Read the model definition and answer for the solid it produces. Units are mm, in the model's axes. Face numbers are marked on the shaded views. A direction names the side the tool comes from. Coordinates: 2 decimals unless noted, no trailing zeros. Write each loop counter-clockwise with the first axis right and the second up, starting at its lowest first coordinate (ties: lowest second). Pieces come first, ordered by that corner, then holes. Notation, with made-up numbers: (41.5, 53) - (70.5, 53) arc R11 cw to (70.5, 61) - close; hole circle Ø7 at (29, -23). An arc over 180 degrees is marked (long way). Use a Markdown table: item, result.
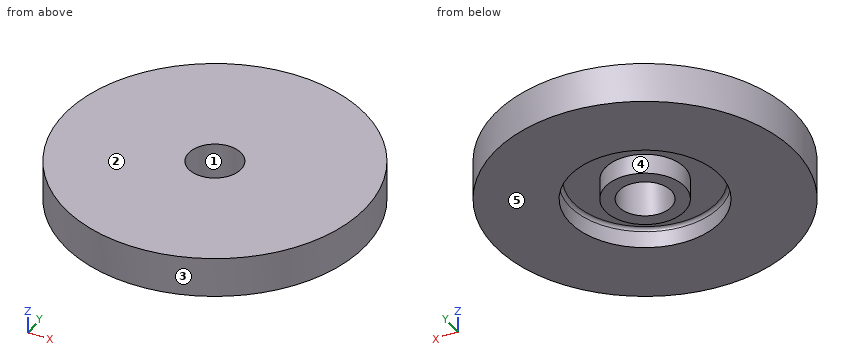
from build123d import *

# Parameters (mm, degrees)
SKETCH_1_R          = 150
SKETCH_1_R_2        = 75
SKETCH_1_R_3        = 38.1
EXTRUDE_1_DEPTH     = 40
SKETCH_1_4_R        = 75
SKETCH_1_4_R_2      = 38.1
CUT_EXTRUDE_1_DEPTH = 20
FILLET_1_R          = 3.2
SCALE_1_SCALE       = 0.4
SKETCH_3_R          = 15.813682359
SKETCH_3_R_2        = 10.461949065
EXTRUDE_2_DEPTH     = 16


with BuildPart() as part:
    # 草图1 → 凸台-拉伸1 (new body)
    # profile 1 of 2: a face of its own
    with BuildSketch(Plane.XY):
        Circle(SKETCH_1_R)
        Circle(SKETCH_1_R_2, mode=Mode.SUBTRACT)
    # profile 2 of 2: a face of its own
    with BuildSketch(Plane.XY):
        Circle(SKETCH_1_R_2)
        Circle(SKETCH_1_R_3, mode=Mode.SUBTRACT)
    extrude(amount=EXTRUDE_1_DEPTH)

    # 草图1<4> → 切除-拉伸1 (cut)
    with BuildSketch(Plane.XY):
        Circle(SKETCH_1_4_R)
        Circle(SKETCH_1_4_R_2, mode=Mode.SUBTRACT)
    extrude(amount=CUT_EXTRUDE_1_DEPTH, mode=Mode.SUBTRACT)

    # 圆角1
    fillet_1_edges = [part.edges().sort_by_distance(p)[0] for p in [
        (-75, 0, 20),
    ]]
    fillet(fillet_1_edges, radius=FILLET_1_R)


with BuildPart() as part_1:
    # 缩放比例1: scaled about (0, 0, 21.099696872)
    add(part.part.scale(SCALE_1_SCALE).moved(Location((0, 0, 12.659818123))))

    # 草图3 → 凸台-拉伸2 (add)
    with BuildSketch(Plane.XY.offset(28.659818123)):
        Circle(SKETCH_3_R)
        Circle(SKETCH_3_R_2, mode=Mode.SUBTRACT)
    extrude(amount=-EXTRUDE_2_DEPTH)


solid = part_1.part
(1) The mould has two halves that part along X. Classify the marked faces 1, 2 and 3: pulls with the +X half, pulls with the -X half, needs draft (parallel to the pull), parting line crosses it, or undercut.
Report:
| item | result |
|---|---|
| face 1 | undercut |
| face 2 | needs draft |
| face 3 | parting line crosses it |
(2) A cutting plane is placed at A-A, the plane x = 0. Write down the section's boundary in (y, z).
Report:
| item | result |
|---|---|
| outline | (-60, 12.66) - (-30, 12.66) - (-30, 19.38) arc R1.28 cw to (-28.72, 20.66) - (-15.81, 20.66) - (-15.81, 12.66) - (-10.46, 12.66) - (-10.46, 28.66) - (-60, 28.66) - close; (10.46, 12.66) - (15.81, 12.66) - (15.81, 20.66) - (28.72, 20.66) arc R1.28 cw to (30, 19.38) - (30, 12.66) - (60, 12.66) - (60, 28.66) - (10.46, 28.66) - close |
(3) Straight lines are drawn through the part: L1, parallel to Y at x = 0, z = 16; L2, parallel to X at y = -14.5, z = 14.25; L3, parallel to Y at x = -16, z = 18.25. For each, find the intervals that lie inside material, in ascending order.
Report:
| item | result |
|---|---|
| L1 | y = -60 to -30, -15.81 to -10.46, 10.46 to 15.81, 30 to 60 |
| L2 | x = -58.22 to -26.26, -6.31 to 6.31, 26.26 to 58.22 |
| L3 | y = -57.83 to -25.38, 25.38 to 57.83 |
(4) A cutting plane is placed at C-C, the plane z = 17.5. Write down the section's boundary in (x, y).
Report:
| item | result |
|---|---|
| outline | circle Ø120 at (0, 0); circle Ø31.63 at (0, 0); hole circle Ø60 at (0, 0); hole circle Ø20.92 at (0, 0) |
(5) For the marked faces 4 and 5, determine the directions among +Z, -Z, +X, -X, +Y, -Y from which every point of the face is accessible in a straight line to the end or side of a thin tool.
Report:
| item | result |
|---|---|
| face 4 | -Z |
| face 5 | -Z, +X, -X, +Y, -Y |
(6) Each of these flat-tipped pins is pushed along its axis until it touches: P1, Ø1, axis at y = 15.5, z = 23.5, coming from the +X side; P2, Ø1, axis at x = -6, z = 20, coming from the -Y side; P3, Ø3, axis at y = 43.5, z = 14.5, coming from the -X side. Where does it stop, or does it pass through?
Report:
| item | result |
|---|---|
| P1 | stops at x = 58.09 |
| P2 | stops at y = -59.75 |
| P3 | stops at x = -42.85 |
(7) A cutting plane is placed at D-D, the plane x = 35. Write down the section's boundary in (y, z), and give its area (3 significant figures).
Report:
| item | result |
|---|---|
| outline | (-48.73, 12.66) - (48.73, 12.66) - (48.73, 28.66) - (-48.73, 28.66) - close |
| area | 1,560 mm² |
